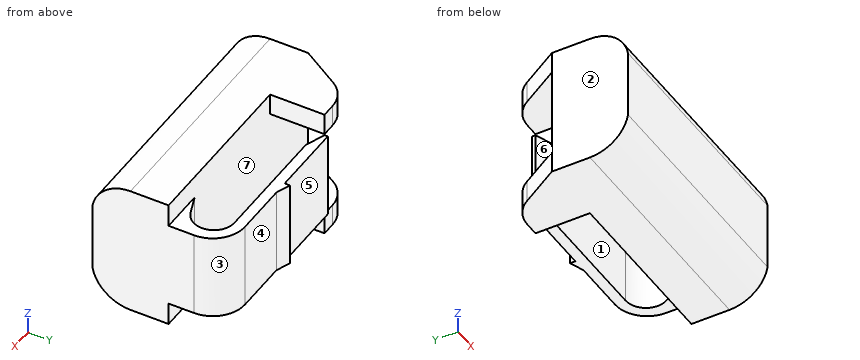
from build123d import *

# Parameters (mm, degrees)
SKETCH1_W                = 22
SKETCH1_H                = 12.2
BOSS_EXTRUDE1_DEPTH      = 7
CUT_EXTRUDE2_REACH       = 28.112
BOSS_EXTRUDE2_DEPTH      = 2
BOSS_EXTRUDE3_DEPTH      = 4
BOSS_EXTRUDE3_DEPTH_BACK = 4


with BuildPart() as part:
    # Sketch1 → Boss-Extrude1 (new body)
    with BuildSketch(Plane(origin=(0, 0, 0), x_dir=(1, 0, 0), z_dir=(0, 1, 0))):
        with Locations((11, 6.1)):
            Rectangle(SKETCH1_W, SKETCH1_H)
    extrude(amount=BOSS_EXTRUDE1_DEPTH)

    # Sketch2 → Cut-Extrude2 (cut, up to next)
    with BuildSketch(Plane(origin=(22, 0, 0), x_dir=(0, 0, -1), z_dir=(1, 0, 0)), mode=Mode.PRIVATE) as cut_extrude2_sk1:
        with BuildLine():
            Line((0, 3.5), (0, 0))
            Line((0, 0), (2.94128103, 0))
            ThreePointArc((2.94128103, 0), (0.832956575, 1.214112093), (0, 3.5))
        make_face()
    cut_extrude2_tool1 = extrude(cut_extrude2_sk1.sketch, amount=-CUT_EXTRUDE2_REACH, mode=Mode.PRIVATE) & part.part
    cut_extrude2 = cut_extrude2_tool1.solids().sort_by_distance((22, 0.790971, -0.742315))[0]
    add(cut_extrude2, mode=Mode.SUBTRACT)

    # Sketch3 → Boss-Extrude2 (add)
    with BuildSketch(Plane(origin=(0, 0, -12.2), x_dir=(-1, 0, 0), z_dir=(0, 0, -1))):
        with BuildLine():
            Line((0, 7), (-6, 7))
            Line((-6, 7), (-6, 12))
            Line((-6, 12), (-4.74458619, 12))
            ThreePointArc((-4.74458619, 12), (-3.278856211, 11.617562918), (-2.186825896, 10.567757085))
            Line((-2.186825896, 10.567757085), (0, 7))
        make_face()
    boss_extrude2 = extrude(amount=-BOSS_EXTRUDE2_DEPTH)

    # Mirror1: Cut-Extrude2, Boss-Extrude2 across plane
    add(cut_extrude2.mirror(Plane.XY.offset(-6.1)), mode=Mode.SUBTRACT)
    add(boss_extrude2.mirror(Plane.XY.offset(-6.1)))

    # Sketch4 → Boss-Extrude3 (add, two sides: drawn at the far end of the back side and taken through both)
    with BuildSketch(Plane.XY.offset(-6.1).offset(-BOSS_EXTRUDE3_DEPTH_BACK)):
        with BuildLine():
            Line((17.895721593, 7), (22, 7))
            Line((22, 7), (22, 9.329014645))
            ThreePointArc((22, 9.329014645), (21.129818536, 11.429818536), (19.029014645, 12.3))
            Line((19.029014645, 12.3), (14.087770897, 12.3))
            Line((14.087770897, 12.3), (12.8, 12.8))
            Line((12.8, 12.8), (12.8, 12.3))
            Line((12.8, 12.3), (6, 12.3))
            Line((6, 12.3), (6, 12))
            Line((6, 12), (7.815685998, 11.327241441))
            Line((7.815685998, 11.327241441), (19.029014645, 11.327241441))
            ThreePointArc((19.029014645, 11.327241441), (20.883632789, 9.783815259), (19.702745838, 7.679705271))
            Line((19.702745838, 7.679705271), (17.895721593, 7))
        make_face()
    extrude(amount=BOSS_EXTRUDE3_DEPTH + BOSS_EXTRUDE3_DEPTH_BACK)


solid = part.part
Work out the finished part from the listing and answer in its coordinate system (mm). Face numbers are marked on the shaded views. A direction names the side the tool comes from. Give positions to 0.01 mm unless a question says otherwise; leave off trailing zeros. Write each loop counter-clockwise with the first axis right and the second up, starting at its lowest first coordinate (ties: lowest second). Pieces come first, ordered by that corner, then holes.
Q1. The part is cut by section D-D on x = 6.25. Give the vertices of the cut face in (y, z), and give its area (3 significant figures).
Answer:
outline: (0, -9.26) arc R3.55 ccw to (3.5, -12.2) - (7, -12.2) - (7, 0) - (3.5, 0) arc R3.55 ccw to (0, -2.94) - close; (11.91, -10.1) - (12.3, -10.1) - (12.3, -2.1) - (11.91, -2.1) - close
area: 83.5 mm2
Q2. For a pull along Y with two mould halves and no side action, classify the marked faces 1, 2 and 3 as released by +Y, released by -Y, zero draft, split by the parting line, or undercut.
Answer:
face 1: undercut
face 2: zero draft
face 3: released by +Y
Q3. The part is cut by section A-A on x = 13.75. Give the vertices of the cut face in (y, z).
Answer:
outline: (0, -9.26) arc R3.55 ccw to (3.5, -12.2) - (7, -12.2) - (7, 0) - (3.5, 0) arc R3.55 ccw to (0, -2.94) - close; (11.33, -10.1) - (12.43, -10.1) - (12.43, -2.1) - (11.33, -2.1) - close
Q4. Straight lines are drawn through the part: L1, parallel to Y at x = 17.5, z = -3.75; L2, parallel to Z at x = 8.5, y = 12.25; L3, parallel to Y at x = 6.25, z = -7.75. For each, find the intervals that lie inside material, in ascending order.
Answer:
L1: y = 0 to 7, 11.33 to 12.3
L2: z = -10.1 to -2.1
L3: y = 0 to 7, 11.91 to 12.3
Q5. The part is cut by section C-C on z = -5.5. Give the vertices of the cut face in (x, y).
Answer:
outline: (0, 0) - (22, 0) - (22, 9.33) arc R2.97 ccw to (19.03, 12.3) - (14.09, 12.3) - (12.8, 12.8) - (12.8, 12.3) - (6, 12.3) - (6, 12) - (7.82, 11.33) - (19.03, 11.33) arc R1.89 cw to (19.7, 7.68) - (17.9, 7) - (0, 7) - close
Q6. The part is cut by section B-B on y = 7.25. Give the vertices of the cut face in (x, z).
Answer:
outline: (0.15, -12.2) - (6, -12.2) - (6, -10.2) - (0.15, -10.2) - close; (0.15, -2) - (6, -2) - (6, 0) - (0.15, 0) - close; (18.56, -10.1) - (22, -10.1) - (22, -2.1) - (18.56, -2.1) - close
Q7. A tool of negligible diameter and unlimited length cuts with its end or side. For the marked faces 4, 5, 6 and 7, from which of +Z, -Z, +X, -X, +Y, -Y can it reach the whole face along a straight path? Write none if from no direction.
Answer:
face 4: +Z, -Z, +X, +Y
face 5: +Z, -Z, -X, +Y
face 6: +Z, -Z, -X
face 7: none
Q8. Given pin 1 (1 mm diameter, centred on y = 9.5, z = -11.5, fed in from +X); pin 2 (4 mm diameter, centred on x = 18, z = -6, fed in from +Y); pin 3 (1 mm diameter, centred on x = 5.5, z = -11.5, fed in from +Y), each flat-ended and moving along its own axis, determine where each tip first touches the part or whether it passes through.
Answer:
pin 1: stops at x = 6
pin 2: stops at y = 12.3
pin 3: stops at y = 12
